Input: part model. Units: mm. Frame: model coordinates. A direction names the side the tool comes from. Give positions to 0.01 mm unless a question says otherwise; leave off trailing zeros. Loops run counter-clockwise (first coordinate to the right, second up) from the corner with the lowest first, then second, coordinate; pieces in that order, holes last. Notation, with made-up numbers: (9, 29.5) - (14, 29.5) arc R14 ccw to (14, 55.5) - close; hole circle Ø9 at (38, 35.25). An arc over 180 degrees is marked (long way). Answer as a JSON object with one key per item and string values. Group by question number.
(1) Section query C-C (x = -3.5). Return loops of the section in (y, z).
(2) Pin query (flat end, axial travel): P1, Ø1.3, axis at y = -7, z = 2.5, coming from the +X side; P2, Ø2, axis at x = -3, z = 2, coming from the -Y side; P3, Ø0.6, axis at x = -12.5, y = 2, coming from the -Z side; P4, Ø4, axis at x = -5, y = 0, coming from the -Z side. Return the tip coordinate at first contact, or that it passes through.
(3) Section query B-B (y = -1.5). Return loops of the section in (x, z), plus the area to 3 significant figures.
(4) Material intervals for L1, parallel to Y at x = -5, z = 1.9; L2, parallel to X at y = 2, z = 1.3; L3, parallel to X at y = -5.5, z = 1.15, sorted ascending.
(5) Access query for faces 4 (the flat face through (-12, 0, 2)), 5 (the flat face through (-9, 0, 4)), 6 (the flat face through (-5, 4.9, 2)), 7 (the flat face through (-5, -4.9, 2)). Directions: +Z, -Z, +X, -X, +Y, -Y. A direction counts if a zero-diameter tool reaches every point of the face in a straight line with its end or side. Return the directions, or none.
(6) Section query A-A (z = 3.25). Return loops of the section in (x, y), plus the area to 3 significant figures.
(7) Mould query, pull axis X, two halves, no side actions, for faces 1 (the flat face through (-11, 0, 1)), 2 (the flat face through (-12.5, -7.5, 2.5)), 3 (the flat face through (-10, 6, 2)). Classes: +X half, -X half, draft (parallel to the pull), parting line (faces both ways), or undercut.
(8) Section query D-D (y = -5.75). Return loops of the section in (x, z).
```python
from build123d import *

# Parameters (mm, degrees)
F1_DEPTH      = 7.5
F1_DEPTH_BACK = 7.5
F2_R          = 2.4
F3_DEPTH      = 4.001
F4_W          = 10
F4_H          = 2.6
F5_DEPTH      = 4.001
F6_R          = 0.5


with BuildPart() as f1:
    # F0 (on Front) → F1 (new body, two sides)
    with BuildSketch(Plane.XZ) as f1_sk:
        Polygon((-11, 0), (0, 0), (0, 4), (-15, 4), (-15, 0), (-13, 0), (-13, 2), (-11, 2), align=None)
    extrude(amount=F1_DEPTH)
    extrude(f1_sk.sketch, amount=-F1_DEPTH_BACK)

    # F2 (on face) → F3 (cut, through all)
    with BuildSketch(Plane.XY.offset(4)):
        with Locations((-5, 0)):
            Circle(F2_R)
    extrude(amount=-F3_DEPTH, mode=Mode.SUBTRACT)

    # F4 (on face) → F5 (cut, through all)
    with BuildSketch(Plane.XY.offset(4)):
        with Locations((-5, 6.2)):
            Rectangle(F4_W, F4_H)
        with Locations((-5, -6.2)):
            Rectangle(F4_W, F4_H)
    extrude(amount=-F5_DEPTH, mode=Mode.SUBTRACT)

    # F6
    f6_edges = [f1.edges().sort_by_distance(p)[0] for p in [
        (-13, 0, 0),
        (-11, 0, 0),
    ]]
    fillet(f6_edges, radius=F6_R)


solid = f1.part
```
Recorded:
{
 "1": {"outline": "(-4.9, 0) - (-1.87, 0) - (-1.87, 4) - (-4.9, 4) - close; (1.87, 0) - (4.9, 0) - (4.9, 4) - (1.87, 4) - close"},
 "2": {"P1": "stops at x = -10", "P2": "stops at y = -4.9", "P3": "stops at z = 2", "P4": "passes through"},
 "3": {"outline": "(-15, 0) - (-13.5, 0) arc R0.5 ccw to (-13, 0.5) - (-13, 2) - (-11, 2) - (-11, 0.5) arc R0.5 ccw to (-10.5, 0) - (-6.87, 0) - (-6.87, 4) - (-15, 4) - close; (-3.13, 0) - (0, 0) - (0, 4) - (-3.13, 4) - close", "area": "40.9 mm^2"},
 "4": {"L1": "y = -4.9 to -2.4, 2.4 to 4.9", "L2": "x = -15 to -13, -11 to -6.33, -3.67 to 0", "L3": "x = -15 to -13, -11 to -10"},
 "5": {"face 4": "-Z, +Y, -Y", "face 5": "+Z, +X, -X, +Y, -Y", "face 6": "+Z, -Z, +X, +Y", "face 7": "+Z, -Z, +X, -Y"},
 "6": {"outline": "(-15, -7.5) - (-10, -7.5) - (-10, -4.9) - (0, -4.9) - (0, 4.9) - (-10, 4.9) - (-10, 7.5) - (-15, 7.5) - close; hole circle Ø4.8 at (-5, 0)", "area": "155 mm^2"},
 "7": {"face 1": "undercut", "face 2": "draft", "face 3": "+X half"},
 "8": {"outline": "(-15, 0) - (-13.5, 0) arc R0.5 ccw to (-13, 0.5) - (-13, 2) - (-11, 2) - (-11, 0.5) arc R0.5 ccw to (-10.5, 0) - (-10, 0) - (-10, 4) - (-15, 4) - close"}
}
